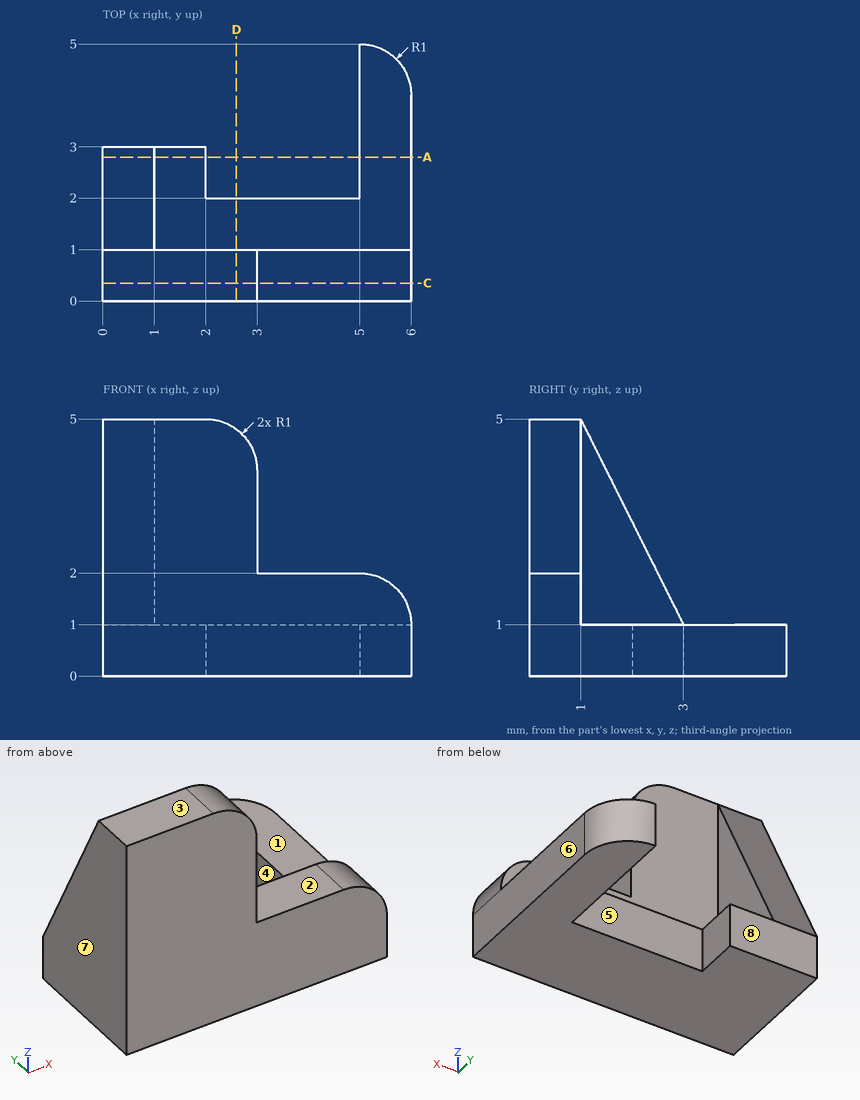
Job drawing, mm, ordinate dimensions from the low corner. One solid piece. A direction names the side the tool comes from. Coordinates: 2 decimals unless noted, no trailing zeros. Write each loop counter-clockwise with the first axis right and the second up, starting at its lowest first coordinate (ties: lowest second). Pieces come first, ordered by that corner, then holes. Notation, with made-up numbers: (80, -3.5) - (96, -3.5) arc R11 ccw to (96, 12.5) - close; hole circle Ø10 at (7.5, -37). An arc over 180 degrees is marked (long way). Use a Markdown table: item, result. Add a question column.
Item 1: 3-axis set-ups, long thin cutter, end or side, ignore diameter. For the marked faces 1, 2, 3 and 4: which of +Z, -Z, +X, -X, +Y, -Y reach the whole face in a straight line?
Item 2: Mould opens along X. For the marked faces 5, 6, 7 and 8 say: pulls with the +X half, pulls with the -X half, needs draft (parallel to the pull), parting line crosses it, or undercut.
Item 3: Band-saw the part on C-C, the plane y = 0.35. Give the cut face in (x, z), and give its area (3 significant figures).
Item 4: Drill centre lines: L1, parallel to X at y = 4, z = 0.65; L2, parallel to Y at x = 1.75, z = 3.25. Where is each one in solid material? Low to high. Write a range as from..to.
Item 5: Band-saw the part on D-D, the plane x = 2.6. Give the cut face in (y, z).
Item 6: Flat gauge pins, fed straight in: pin 1 (0.5 mm diameter, centred on x = 4, y = 0.5, fed in from +Z); pin 2 (1 mm diameter, centred on x = 2, z = 2.5, fed in from +Y); pin 3 (0.5 mm diameter, centred on y = 0.5, z = 3, fed in from +X); pin 4 (3 mm diameter, centred on x = 2.5, y = 0.5, fed in from +Z). Where does each tip first touch, or does it go through?
Item 7: Band-saw the part on A-A, the plane y = 2.8. Give the cut face in (x, z), and give its area (3 significant figures).
Numbers:
| question | item | result |
|---|---|---|
| 1 | face 1 | +Z, +X, +Y |
| 1 | face 2 | +Z, +X, +Y, -Y |
| 1 | face 3 | +Z, +X, -X, +Y, -Y |
| 1 | face 4 | +Z, -Z, +Y |
| 2 | face 5 | undercut |
| 2 | face 6 | pulls with the +X half |
| 2 | face 7 | pulls with the -X half |
| 2 | face 8 | needs draft |
| 3 | outline | (0, 0) - (6, 0) - (6, 1) arc R1 ccw to (5, 2) - (3, 2) - (3, 4) arc R1 ccw to (2, 5) - (0, 5) - close |
| 3 | area | 20.6 mm2 |
| 4 | L1 | 5..6 |
| 4 | L2 | 0..1 |
| 5 | outline | (0, 0) - (2, 0) - (2, 1) - (1, 1) - (1, 4.8) - (0, 4.8) - close |
| 6 | pin 1 | z = 2 |
| 6 | pin 2 | y = 1 |
| 6 | pin 3 | x = 3 |
| 6 | pin 4 | z = 5 |
| 7 | outline | (0, 0) - (2, 0) - (2, 1) - (1, 1) - (1, 1.4) - (0, 1.4) - close; (5, 0) - (6, 0) - (6, 1) - (5, 1) - close |
| 7 | area | 3.40 mm2 |
